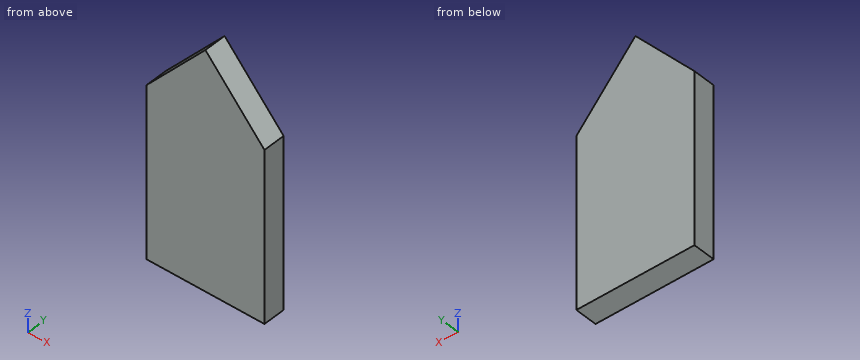
```python
from build123d import *

# Parameters (mm, degrees)
F0_W     = 101.6
F0_H     = 203.2
F1_DEPTH = 19.05
F3_DEPTH = 19.051


with BuildPart() as f1:
    # F0 (on Front) → F1 (new body)
    with BuildSketch(Plane.XZ):
        Rectangle(F0_W, F0_H)
    extrude(amount=F1_DEPTH)

    # F2 (on face) → F3 (cut, through all)
    with BuildSketch(Plane.XZ.offset(19.05)):
        Polygon((-50.8, 44.803873), (0, 101.6), (-50.8, 101.6), align=None)
        Polygon((50.8, 101.6), (0, 101.6), (50.8, 44.803873), align=None)
    extrude(amount=-F3_DEPTH, mode=Mode.SUBTRACT)


solid = f1.part
```
Work out the finished part from the listing and answer in its coordinate system (mm). Round coordinates to 2 decimals unless told otherwise and drop trailing zeros. Order: outer loops, then holes, each group sorted by start corner. A loop starts at its lowest first (then second) coordinate and runs counter-clockwise, first axis right, second up.
Q1. A cutting plane is placed at A-A, the plane y = -6.5. Determine the outline of the cut face in (x, z), then the cut area to 3 significant figures.
Solution:
outline: (-50.8, -101.6) - (50.8, -101.6) - (50.8, 44.8) - (0, 101.6) - (-50.8, 44.8) - close
area: 17,800 mm2
Q2. Given pin 1 Ø8 at (x, y) = (-22.5, -13.5) entering from +Z; pin 2 Ø4 at (x, y) = (33.5, -15) entering from +Z, each flat-ended and moving along its own axis, determine where each tip first touches the part or whether it passes through.
Solution:
pin 1: stops at z = 80.92
pin 2: stops at z = 66.38
Q3. A cutting plane is placed at B-B, the plane x = -23.5. Determine the outline of the cut face in (y, z).
Solution:
outline: (-19.05, -101.6) - (0, -101.6) - (0, 75.33) - (-19.05, 75.33) - close
Q4. A cutting plane is placed at C-C, the plane x = -40. Determine the outline of the cut face in (y, z), then the cut area to 3 significant figures.
Solution:
outline: (-19.05, -101.6) - (0, -101.6) - (0, 56.88) - (-19.05, 56.88) - close
area: 3,020 mm2
Q5. Find the intervals of material crossed by line 1 along Z through (x, y) = (17, -16); line 2 along Z through (x, y) = (-44.5, -2.5); line 3 along X through (y, z) = (-15, 90.5), in increasing order.
Solution:
line 1: z = -101.6 to 82.59
line 2: z = -101.6 to 51.85
line 3: x = -9.93 to 9.93
